The model under review builds one solid part; all positions refer to its coordinate system, in mm. Coordinates: 2 decimals unless noted, no trailing zeros. Order: outer loops, then holes, each group sorted by start corner. A loop starts at its lowest first (then second) coordinate and runs counter-clockwise, first axis right, second up.
```python
from build123d import *

# Parameters (mm, degrees)
SALIENTE_EXTRUIR1_DEPTH = 2
CROQUIS4_R              = 1.75
CORTAR_EXTRUIR1_DEPTH   = 2
REDONDEO1_R             = 10
REDONDEO2_R             = 8


with BuildPart() as part:
    # Croquis2 → Saliente-Extruir1 (new body)
    with BuildSketch(Plane.XY):
        Polygon((0, 40), (0, 0), (19.4, 0), (19.4, 10.5), (1.59, 10.5), (1.59, 14.5), (42.21, 14.5), (42.21, 10.5), (24.4, 10.5), (24.4, 0), (43.8, 0), (43.8, 40), (24.4, 40), (24.4, 29.5), (42.21, 29.5), (42.21, 25.5), (1.59, 25.5), (1.59, 29.5), (19.4, 29.5), (19.4, 40), align=None)
    extrude(amount=SALIENTE_EXTRUIR1_DEPTH)

    # Croquis4 → Cortar-Extruir1 (cut)
    with BuildSketch(Plane.XY.offset(2)):
        with Locations((15, 35)):
            Circle(CROQUIS4_R)
        with Locations((15, 3.5)):
            Circle(CROQUIS4_R)
        with Locations((33.8, 35)):
            Circle(CROQUIS4_R)
        with Locations((33.8, 3.5)):
            Circle(CROQUIS4_R)
    extrude(amount=-CORTAR_EXTRUIR1_DEPTH, mode=Mode.SUBTRACT)

    # Redondeo1
    redondeo1_edges = [part.edges().sort_by_distance(p)[0] for p in [
        (43.8, 40, 1),
        (43.8, 0, 1),
    ]]
    fillet(redondeo1_edges, radius=REDONDEO1_R)

    # Redondeo2
    redondeo2_edges = [part.edges().sort_by_distance(p)[0] for p in [
        (0, 0, 1),
        (0, 40, 1),
    ]]
    fillet(redondeo2_edges, radius=REDONDEO2_R)


solid = part.part
```
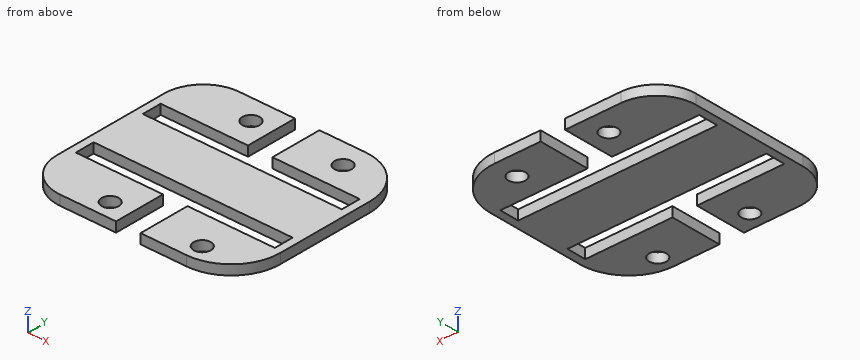
(1) We need section C-C, the plane y = 34.5. Write out the cut boundary in (x, z), and give its area (3 significant figures).
A:
outline: (0.4, 0) - (13.32, 0) - (13.32, 2) - (0.4, 2) - close; (16.68, 0) - (19.4, 0) - (19.4, 2) - (16.68, 2) - close; (24.4, 0) - (32.12, 0) - (32.12, 2) - (24.4, 2) - close; (35.48, 0) - (42.73, 0) - (42.73, 2) - (35.48, 2) - close
area: 61.2 mm2
(2) We need section A-A, the plane z = 0.6. Write out the cut boundary in (x, y).
A:
outline: (0, 8) arc R8 ccw to (8, 0) - (19.4, 0) - (19.4, 10.5) - (1.59, 10.5) - (1.59, 14.5) - (42.21, 14.5) - (42.21, 10.5) - (24.4, 10.5) - (24.4, 0) - (33.8, 0) arc R10 ccw to (43.8, 10) - (43.8, 30) arc R10 ccw to (33.8, 40) - (24.4, 40) - (24.4, 29.5) - (42.21, 29.5) - (42.21, 25.5) - (1.59, 25.5) - (1.59, 29.5) - (19.4, 29.5) - (19.4, 40) - (8, 40) arc R8 ccw to (0, 32) - close; hole circle Ø3.5 at (15, 3.5); hole circle Ø3.5 at (15, 35); hole circle Ø3.5 at (33.8, 3.5); hole circle Ø3.5 at (33.8, 35)
(3) For pin 1 Ø4.5 at (x, y) = (15, 3.5) entering from -Z; pin 2 Ø0.6 at (y, z) = (33, 1.5) entering from +X; pin 3 Ø1 at (y, z) = (33.5, 1.5) entering from -X, all flat-tipped, find the tip position at first contact; note any pin that passes through.
A:
pin 1: stops at z = 0
pin 2: stops at x = 43.43
pin 3: stops at x = 0.06
(4) We need section D-D, the plane x = 15. Write out the cut boundary in (y, z).
A:
outline: (0, 0) - (1.75, 0) - (1.75, 2) - (0, 2) - close; (5.25, 0) - (10.5, 0) - (10.5, 2) - (5.25, 2) - close; (14.5, 0) - (25.5, 0) - (25.5, 2) - (14.5, 2) - close; (29.5, 0) - (33.25, 0) - (33.25, 2) - (29.5, 2) - close; (36.75, 0) - (40, 0) - (40, 2) - (36.75, 2) - close
(5) Wall thickness on probe 1 along Y at (x, z) = (18.5, 1); probe 2 along Y at (x, z) = (15, 0.9); probe 3 along Y at (x, z) = (41, 0.6): over which ranges is each line inside the solid? List them lowest first.
A:
probe 1: y = 0 to 10.5, 14.5 to 25.5, 29.5 to 40
probe 2: y = 0 to 1.75, 5.25 to 10.5, 14.5 to 25.5, 29.5 to 33.25, 36.75 to 40
probe 3: y = 3.06 to 10.5, 14.5 to 25.5, 29.5 to 36.94
(6) We need section B-B, the plane x = 28.5. Write out the cut boundary in (y, z), and give its area (3 significant figures).
A:
outline: (0, 0) - (10.5, 0) - (10.5, 2) - (0, 2) - close; (14.5, 0) - (25.5, 0) - (25.5, 2) - (14.5, 2) - close; (29.5, 0) - (40, 0) - (40, 2) - (29.5, 2) - close
area: 64.0 mm2
